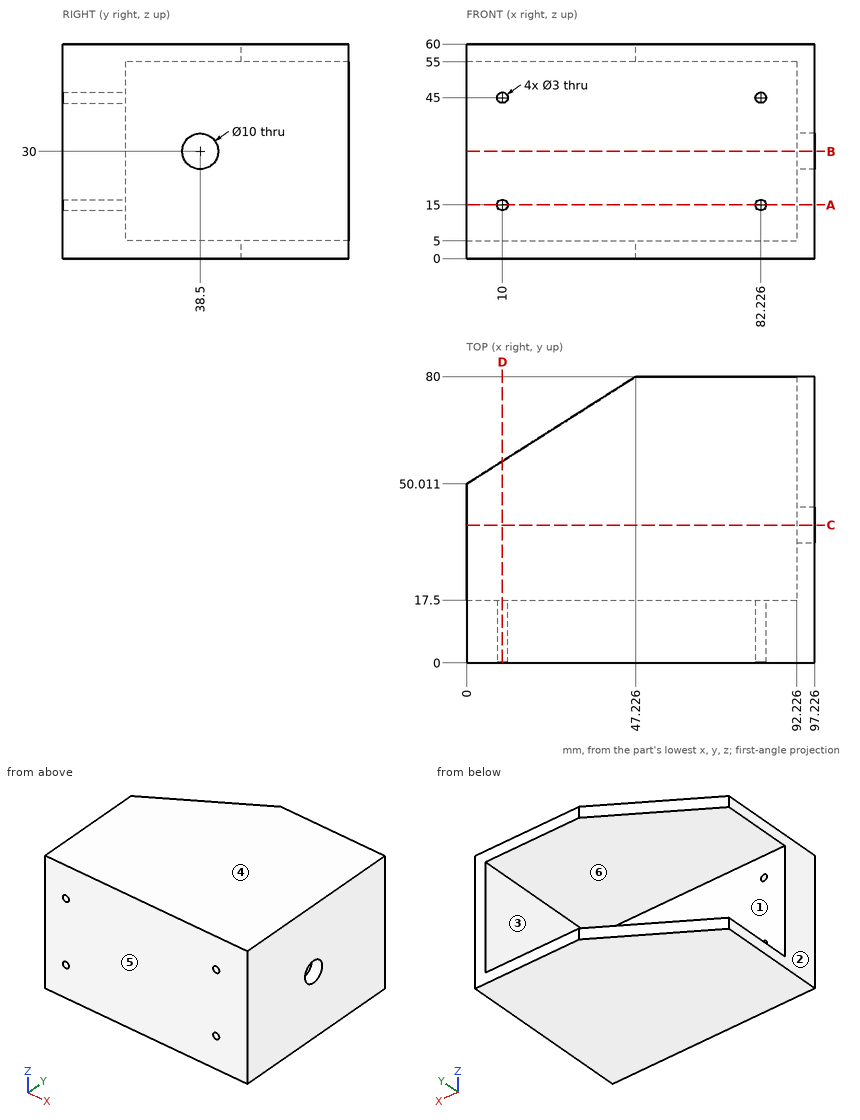
Check sheet for the drawn part. Datum: minimum x, y, z corner. Units: mm. A direction names the side the tool comes from. Round coordinates to 2 decimals unless told otherwise and drop trailing zeros. Loops run counter-clockwise (first coordinate to the right, second up) from the corner with the lowest first, then second, coordinate; pieces in that order, holes last. Notation, with made-up numbers: M 44.5,-5 L 68.5,-5 A29 cw 68.5,24 Z; hole C 49.25,43 d2. An arc over 180 degrees is marked long. Write each question's results on one line, items separated by ' | '.
1) Section check B-B on z = 30. Record the boundary of the cut face in (x, y).
Checks:
outline: M 0,0 L 97.23,0 L 97.23,33.5 L 92.23,33.5 L 92.23,17.5 L 0,17.5 Z; M 92.23,43.5 L 97.23,43.5 L 97.23,80 L 92.23,80 Z
2) Scan lines: L1, parallel to Z at x = 10, y = 10.5; L2, parallel to Z at x = 23, y = 34; L3, parallel to Y at x = 8.5, z = 31.5. Record each from-to range of solid material in increasing order. Write a range as from..to.
Checks:
L1: z = 0..13.5, 16.5..43.5, 46.5..60 | L2: z = 0..5, 55..60 | L3: y = 0..17.5
3) Gauge pin test, flat ends, axial feed: P1, Ø5, axis at x = 83, y = 11.5, coming from the -Z side; P2, Ø4, axis at x = 10, z = 45, coming from the +Y side; P3, Ø1, axis at y = 29, z = 50, coming from the -X side. Record the tip position at first contact, or that the pin passes through.
Checks:
P1: stops at z = 0 | P2: stops at y = 17.5 | P3: stops at x = 92.23
4) Section check D-D on x = 10. Record the boundary of the cut face in (y, z), then the cut area to 3 significant figures.
Checks:
outline: M 0,0 L 56.36,0 L 56.36,5 L 17.5,5 L 17.5,13.5 L 0,13.5 Z; M 0,16.5 L 17.5,16.5 L 17.5,43.5 L 0,43.5 Z; M 0,46.5 L 17.5,46.5 L 17.5,55 L 56.36,55 L 56.36,60 L 0,60 Z | area: 1,330 mm2
5) Mould release check, pull along Z, two halves, no side actions. Record for the marked faces 1, 2, 3 and 4: released by +Z, released by -Z, zero draft, split by the parting line, or undercut.
Checks:
face 1: undercut | face 2: zero draft | face 3: undercut | face 4: released by +Z
6) Access from +Z, -Z, +X, -X, +Y, -Y to the whole of each face (thin tool, end or side, straight path). Record for the marked faces 5 and 6.
Checks:
face 5: +Z, -Z, +X, -X, -Y | face 6: -X, +Y
7) Section check A-A on z = 15. Record the boundary of the cut face in (x, y), then the cut area to 3 significant figures.
Checks:
outline: M 0,0 L 8.5,0 L 8.5,17.5 L 0,17.5 Z; M 11.5,0 L 80.73,0 L 80.73,17.5 L 11.5,17.5 Z; M 83.73,0 L 97.23,0 L 97.23,80 L 92.23,80 L 92.23,17.5 L 83.73,17.5 Z | area: 1,910 mm2
8) Section check C-C on y = 38.5. Record the boundary of the cut face in (x, z).
Checks:
outline: M 0,0 L 97.23,0 L 97.23,25 L 92.23,25 L 92.23,5 L 0,5 Z; M 0,55 L 92.23,55 L 92.23,35 L 97.23,35 L 97.23,60 L 0,60 Z
